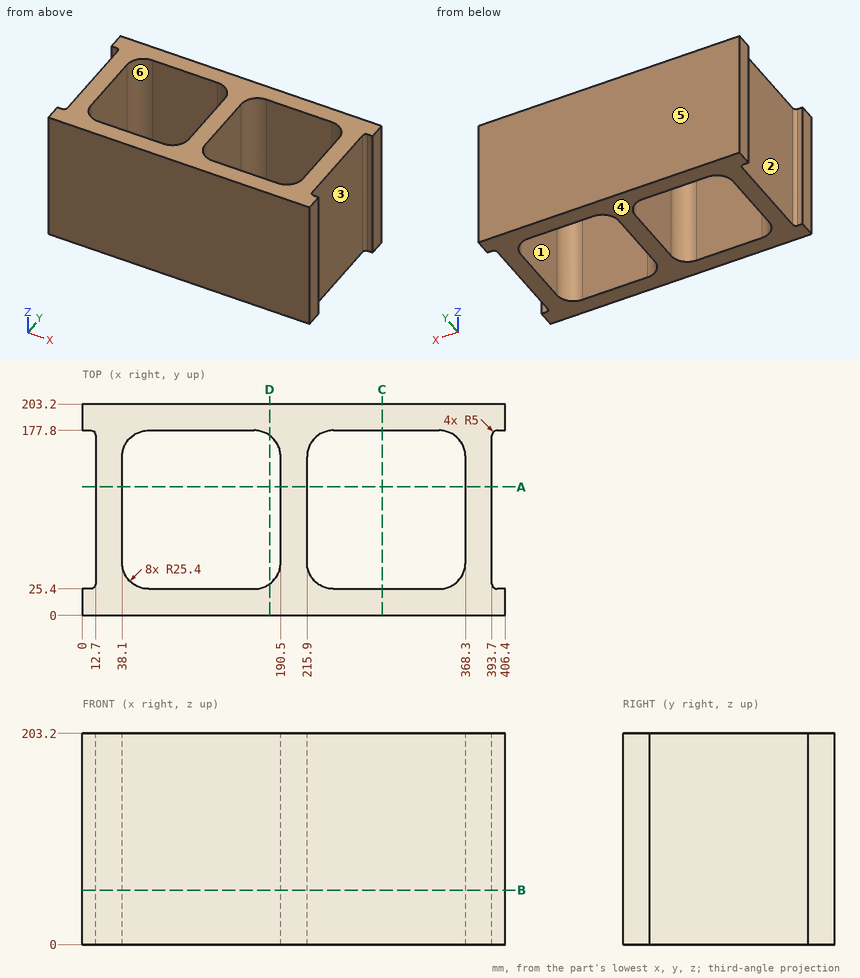
Could you check a few things on this drawing? It's one solid part, dimensions in mm from its lowest x, y, z. A direction names the side the tool comes from. Coordinates: 2 decimals unless noted, no trailing zeros. Order: outer loops, then holes, each group sorted by start corner. A loop starts at its lowest first (then second) coordinate and runs counter-clockwise, first axis right, second up. Notation, with made-up numbers: (79.5, 45) -> (101.5, 45) arc R5 cw to (101.5, 49) -> close; hole circle Ø7 at (12, 68.25). An arc over 180 degrees is marked (long way). Answer in a Markdown table with one row per item.
(1) Thinking about a two-plate mould opening in Y: for the marked faces 4, 5 and 6, which applies, +Y half, -Y half, draft (parallel to the pull), parting line (faces both ways), or undercut?
Answer key:
| item | result |
|---|---|
| face 4 | draft |
| face 5 | +Y half |
| face 6 | undercut |
(2) Please list where these lines run through material, in increasing order: probe 1 along X at (y, z) = (151, 136.5); probe 2 along Y at (x, z) = (123.5, 178); probe 3 along X at (y, z) = (172, 79.5).
Answer key:
| item | result |
|---|---|
| probe 1 | 12.7 to 38.1, 190.5 to 215.9, 368.3 to 393.7 |
| probe 2 | 0 to 25.4, 177.8 to 203.2 |
| probe 3 | 12.7 to 47.34, 181.26 to 225.14, 359.06 to 393.7 |
(3) Will these pins go through, and if not, where does the flat tip stop? pin 1 Ø6 at (x, z) = (337.5, 32.5) entering from -Y; pin 2 Ø1 at (y, z) = (146.5, 148) entering from -X.
Answer key:
| item | result |
|---|---|
| pin 1 | y = 0 |
| pin 2 | x = 12.7 |
(4) I want a section at A-A on y = 123.5. List the corners of the cut face in (x, z) for me.
Answer key:
| item | result |
|---|---|
| outline | (12.7, 0) -> (38.1, 0) -> (38.1, 203.2) -> (12.7, 203.2) -> close; (190.5, 0) -> (215.9, 0) -> (215.9, 203.2) -> (190.5, 203.2) -> close; (368.3, 0) -> (393.7, 0) -> (393.7, 203.2) -> (368.3, 203.2) -> close |
(5) I want a section at B-B on z = 52.5. Count the separate pieces of the cut face and the enclosed holes in it, then the cut area to 3 significant figures.
Answer key:
| item | result |
|---|---|
| separate pieces | 1 |
| enclosed holes | 2 |
| area | 33,400 mm^2 |
(6) I want a section at D-D on x = 180. List the corners of the cut face in (y, z) for me.
Answer key:
| item | result |
|---|---|
| outline | (0, 0) -> (30.23, 0) -> (30.23, 203.2) -> (0, 203.2) -> close; (172.97, 0) -> (203.2, 0) -> (203.2, 203.2) -> (172.97, 203.2) -> close |
(7) I want a section at C-C on x = 288. List the corners of the cut face in (y, z) for me, then the cut area to 3 significant figures.
Answer key:
| item | result |
|---|---|
| outline | (0, 0) -> (25.4, 0) -> (25.4, 203.2) -> (0, 203.2) -> close; (177.8, 0) -> (203.2, 0) -> (203.2, 203.2) -> (177.8, 203.2) -> close |
| area | 10,300 mm^2 |
(8) On a 3-axis mill with a long thin cutter (end or side, diameter ignored), from which of +Z, -Z, +X, -X, +Y, -Y can I reach the whole of each face in a straight line? I mean the marked faces 1, 2 and 3. Say none if no direction works.
Answer key:
| item | result |
|---|---|
| face 1 | +Z, -Z |
| face 2 | +Z, -Z, -X |
| face 3 | +Z, -Z, +X |
